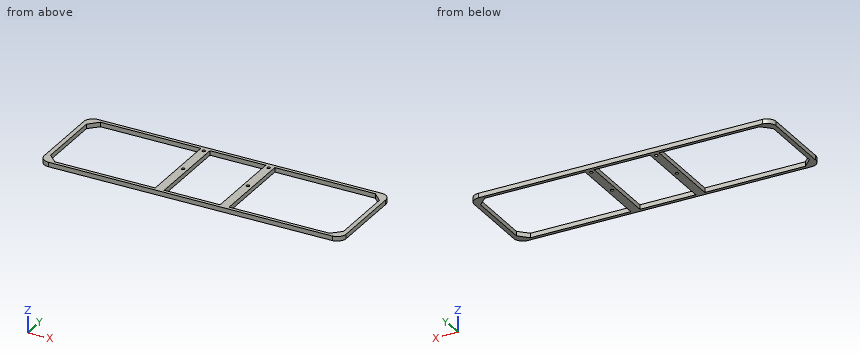
from build123d import *

# Parameters (mm, degrees)
SKETCH1_W           = 335
SKETCH1_H           = 100
SKETCH1_R           = 1.75
SKETCH1_W_2         = 62
SKETCH1_H_2         = 92.5
SKETCH1_W_3         = 121.5
BOSS_EXTRUDE1_DEPTH = 5
FILLET1_R           = 10
CHAMFER1_SIZE       = 10


with BuildPart() as part:
    # Sketch1 → Boss-Extrude1 (new body)
    with BuildSketch(Plane.XY):
        Rectangle(SKETCH1_W, SKETCH1_H)
        with Locations((-36, 43)):
            Circle(SKETCH1_R, mode=Mode.SUBTRACT)
        with Locations((36, 43)):
            Circle(SKETCH1_R, mode=Mode.SUBTRACT)
        with Locations((36, 1)):
            Circle(SKETCH1_R, mode=Mode.SUBTRACT)
        with Locations((-36, 1)):
            Circle(SKETCH1_R, mode=Mode.SUBTRACT)
        Rectangle(SKETCH1_W_2, SKETCH1_H_2, mode=Mode.SUBTRACT)
        with Locations((-101.75, 0)):
            Rectangle(SKETCH1_W_3, SKETCH1_H_2, mode=Mode.SUBTRACT)
        with Locations((101.75, 0)):
            Rectangle(SKETCH1_W_3, SKETCH1_H_2, mode=Mode.SUBTRACT)
    extrude(amount=-BOSS_EXTRUDE1_DEPTH)

    # Fillet1
    fillet1_edges = [part.edges().sort_by_distance(p)[0] for p in [
        (167.5, -50, -2.5),
        (-167.5, -50, -2.5),
        (-167.5, 50, -2.5),
        (167.5, 50, -2.5),
    ]]
    fillet(fillet1_edges, radius=FILLET1_R)

    # Chamfer1
    chamfer1_edges = [part.edges().sort_by_distance(p)[0] for p in [
        (162.5, 46.25, -2.5),
        (162.5, -46.25, -2.5),
        (-162.5, -46.25, -2.5),
        (-162.5, 46.25, -2.5),
    ]]
    chamfer(chamfer1_edges, length=CHAMFER1_SIZE)


solid = part.part
Work out the finished part from the listing and answer in its coordinate system (mm). Give positions to 0.01 mm unless a question says otherwise; leave off trailing zeros. Order: outer loops, then holes, each group sorted by start corner. A loop starts at its lowest first (then second) coordinate and runs counter-clockwise, first axis right, second up. Notation, with made-up numbers: M 25.25,76 L 40.25,76 A19 ccw 40.25,85 Z; hole C -32.5,58.25 d7. An arc over 180 degrees is marked long. Return JSON: item names as keys, results as strings.
Q1. Find section B-B, the plane x = 106. Write down the section's boundary in (y, z).
Answer below:
{"outline": "M -50,-5 L -46.25,-5 L -46.25,0 L -50,0 Z; M 46.25,-5 L 50,-5 L 50,0 L 46.25,0 Z"}
Q2. Find the intervals of material crossed by line 1 along Y through (x, z) = (-36, -1.95); line 2 along X through (y, z) = (-19, -1.75); line 3 along Y through (x, z) = (-68, -2.7), in increasing order. Write a range as [from, to].
Answer below:
{"line 1": "y = [-50, -0.75], [2.75, 41.25], [44.75, 50]", "line 2": "x = [-167.5, -162.5], [-41, -31], [31, 41], [162.5, 167.5]", "line 3": "y = [-50, -46.25], [46.25, 50]"}
Q3. Find section C-C, the plane y = -6. Write down the section's boundary in (x, z), and give its area (3 significant figures).
Answer below:
{"outline": "M -167.5,-5 L -162.5,-5 L -162.5,0 L -167.5,0 Z; M -41,-5 L -31,-5 L -31,0 L -41,0 Z; M 31,-5 L 41,-5 L 41,0 L 31,0 Z; M 162.5,-5 L 167.5,-5 L 167.5,0 L 162.5,0 Z", "area": "150 mm^2"}
Q4. Find section A-A, the plane z = -2.45. Write down the section's boundary in (x, y), and give its area (3 significant figures).
Answer below:
{"outline": "M -167.5,-40 A10 ccw -157.5,-50 L 157.5,-50 A10 ccw 167.5,-40 L 167.5,40 A10 ccw 157.5,50 L -157.5,50 A10 ccw -167.5,40 Z; hole M -162.5,-36.25 L -152.5,-46.25 L -41,-46.25 L -41,46.25 L -152.5,46.25 L -162.5,36.25 Z; hole C -36,1 d3.5; hole C -36,43 d3.5; hole M -31,-46.25 L 31,-46.25 L 31,46.25 L -31,46.25 Z; hole C 36,1 d3.5; hole C 36,43 d3.5; hole M 41,-46.25 L 152.5,-46.25 L 162.5,-36.25 L 162.5,36.25 L 152.5,46.25 L 41,46.25 Z", "area": "5,360 mm^2"}
Q5. This flat-tipped pin is pushed along its axis until it touches: pin 1 (4.5 mm diameter, centred on x = 36, y = 43, fed in from -Z). Where does it stop, or does it pass through?
Answer below:
{"pin 1": "stops at z = -5"}
